Autodesk Inventor part; units mm, degrees
ref_plane "YZ Plane" through (0, 0, 0) normal (1, 0, 0) x (0, 1, 0)
ref_plane "XZ Plane" through (0, 0, 0) normal (0, 1, 0) x (-1, 0, 0)
ref_plane "XY Plane" through (0, 0, 0) normal (0, 0, 1) x (1, 0, 0)
sketch "Sketch1" plane through (0, 0, 0) normal (0, 1, 0) x (-1, 0, 0)
  line L0 (0, 0) -> (279.4, 0)
  line L1 (279.4, 0) -> (279.4, -44.577)
  line L2 (279.4, -44.577) -> (0, -44.577)
  line L3 (0, -44.577) -> (0, 0)
  dimension "d0" = 279.4
  dimension "d1" = 44.577
extrude "Extrusion1" add sketch "Sketch1" along normal blind 3.175
sketch "Sketch2" plane through (0, 3.175, 0) normal (0, 1, 0) x (1, 0, 0)
  line L0 (-279.4, 0) -> (0, 0)
  line L1 (-279.4, 0) -> (0, 0)
  line L2 (0, 0) -> (0, 3.175)
  line L3 (0, 3.175) -> (-279.4, 3.175)
  line L4 (-279.4, 3.175) -> (-279.4, 0)
  dimension "d4" = 279.4
  dimension "d5" = 3.175
extrude "Extrusion2" add sketch "Sketch2" along normal blind 25.4
sketch "Sketch3" plane through (0, 3.175, 0) normal (0, 1, 0) x (1, 0, 0)
  line L0 (0, 3.175) -> (0, 44.577) construction
  line L1 (0, 44.577) -> (-279.4, 44.577) construction
  line L2 (-139.7, 44.577) -> (-139.7, 3.175) construction
  line L3 (0, 44.577) -> (-30.8102, 44.577) construction
  line L4 (-30.8102, 44.577) -> (-30.8102, 20.574) construction
  circle A0 centre (-30.8102, 20.574) radius 2.5797
  line L5 (-30.8102, 20.574) -> (-15.2628, 31.5822) construction
  circle A1 centre (-15.2628, 31.5822) radius 2.5797
  point P0 (0, 0)
extrude "Extrusion3" cut sketch "Sketch3" against normal blind 25.4
sketch "Sketch4" plane through (0, 3.175, 0) normal (0, 1, 0) x (1, 0, 0)
  line L0 (-279.4, 44.577) -> (-279.4, 3.175) construction
  line L1 (-279.4, 23.876) -> (-266.7, 23.876) construction
  circle A0 centre (-266.7, 23.876) radius 2.5797
  point P0 (0, 0)
  dimension "d26" = 12.7
  dimension "d27" = 5.1594
extrude "Extrusion4" cut sketch "Sketch4" against normal blind 25.4
properties part number "angle iron with  holes 1"
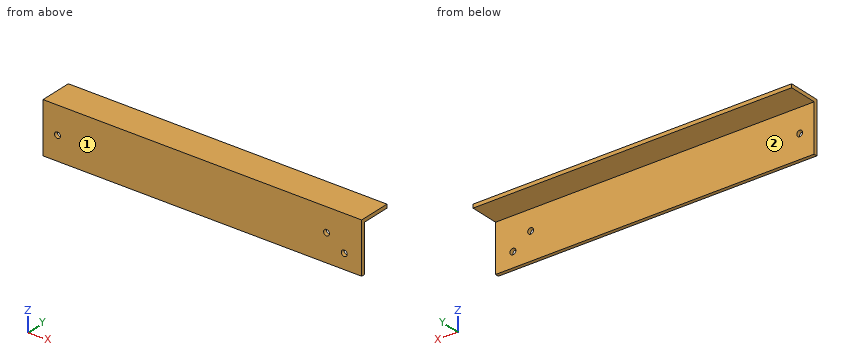
Model file for the job. Use its own axes, mm. Face numbers are marked on the shaded views. A direction names the side the tool comes from. Coordinates: 2 decimals unless noted, no trailing zeros. Loops run counter-clockwise (first coordinate to the right, second up) from the corner with the lowest first, then second, coordinate; pieces in that order, holes last. Notation, with made-up numbers: M 55.5,-30 L 74.5,-30 A18 cw 74.5,-1 Z; hole C -31.75,74 d8. An arc over 180 degrees is marked long. Use CSV: the item, a comma, the result in double quotes. Start each with the question number.
1. Tool access for the marked faces 1 and 2: list every direction of +Z, -Z, +X, -X, +Y, -Y with a clear straight run to the whole face (end or side of a thin tool).
2. Band-saw the part on C-C, the plane x = -167. List the corners of the cut face in (y, z) (3 decimals), then the cut area to 3 significant figures.
3. Probe probe 1 along Z at (x, y) = (-266.7, 0.7); probe 2 along Z at (x, y) = (-104, 20.75) (3 decimals); probe 3 along Y at (x, z) = (-147.5, -4) (3 decimals). List the from-to ranges inside material, lowest first. Write a range as [from, to].
4. Band-saw the part on D-D, the plane z = -7. List the corners of the cut face in (x, y) (3 decimals), then the cut area to 3 significant figures.
5. Band-saw the part on B-B, the plane y = 20.5. List the corners of the cut face in (x, z) (3 decimals), then the cut area to 3 significant figures.
6. Band-saw the part on A-A, the plane x = -266.7. List the corners of the cut face in (y, z) (3 decimals), then the cut area to 3 significant figures.
7. Flat gauge pins, fed straight in: pin 1 (6 mm diameter, centred on x = -172.5, y = 8.5, fed in from +Z); pin 2 (8 mm diameter, centred on x = -37.5, z = -15.5, fed in from +Y) (3 decimals); pin 3 (6 mm diameter, centred on x = -214.5, y = 17, fed in from -Z) (3 decimals). Where does each tip first touch, or does it go through?
Entries:
1,face 1,"+Z, -Z, +X, -X, -Y"
1,face 2,"-Z, +X, -X, +Y"
2,outline,"M 0,-44.577 L 3.175,-44.577 L 3.175,-3.175 L 28.575,-3.175 L 28.575,0 L 0,0 Z"
2,area,"222 mm2"
3,probe 1,"z = [-44.58, -26.46], [-21.3, 0]"
3,probe 2,"z = [-3.175, 0]"
3,probe 3,"y = [0, 3.175]"
4,outline,"M -279.4,0 L 0,0 L 0,3.175 L -279.4,3.175 Z"
4,area,"887 mm2"
5,outline,"M -279.4,-3.175 L 0,-3.175 L 0,0 L -279.4,0 Z"
5,area,"887 mm2"
6,outline,"M 0,-44.577 L 3.175,-44.577 L 3.175,-26.456 L 0,-26.456 Z; M 0,-21.296 L 3.175,-21.296 L 3.175,-3.175 L 28.575,-3.175 L 28.575,0 L 0,0 Z"
6,area,"206 mm2"
7,pin 1,"stops at z = 0"
7,pin 2,"stops at y = 3.175"
7,pin 3,"stops at z = -3.175"
